Design review of the part built by this model. Coordinates are the model's own, in mm. Face numbers are marked on the shaded views. A direction names the side the tool comes from. Give positions to 0.01 mm unless a question says otherwise; leave off trailing zeros. Order: outer loops, then holes, each group sorted by start corner. A loop starts at its lowest first (then second) coordinate and runs counter-clockwise, first axis right, second up. Notation, with made-up numbers: (11.5, 53.5) - (48.5, 53.5) arc R29 ccw to (48.5, 85.5) - close; hole circle Ø6 at (-1.5, 80). An arc over 180 degrees is marked (long way). Write each question's results on one line, items separated by ' | '. Start each with the question number.
```python
from build123d import *
from build123d import SkipClean  # not in build123d's __all__

# Parameters (mm, degrees)
F0_R     = 50.8
F0_R_2   = 6.35
F0_R_3   = 19.05
F1_DEPTH = 12.7
F2_R     = 25.4
F3_DEPTH = 76.2
F4_R     = 50.8
F4_R_2   = 6.35
F4_R_3   = 19.05
F5_DEPTH = 12.7
F6_R     = 19.05
F7_DEPTH = 76.2


# Not quite as in the source:
# - a feature names something its author has since deleted; it is built from what else it names


with BuildPart() as f1:
    # F0 (on Front) → F1 (new body)
    with BuildSketch(Plane.XZ):
        Circle(F0_R)
        with Locations((-28.575, -28.575)):
            Circle(F0_R_2, mode=Mode.SUBTRACT)
        Circle(F0_R_3, mode=Mode.SUBTRACT)
        with Locations((28.575, -28.575)):
            Circle(F0_R_2, mode=Mode.SUBTRACT)
        with Locations((-28.575, 28.575)):
            Circle(F0_R_2, mode=Mode.SUBTRACT)
        with Locations((28.575, 28.575)):
            Circle(F0_R_2, mode=Mode.SUBTRACT)
    extrude(amount=F1_DEPTH)

    # F2 (on face) → F3 (join)
    with BuildSketch(Plane(origin=(0, 0, 0), x_dir=(-1, 0, 0), z_dir=(0, 1, 0))):
        Circle(F2_R)
    extrude(amount=F3_DEPTH)

    # F4 (on face) → F5 (join)
    with BuildSketch(Plane(origin=(0, 76.2, 0), x_dir=(-1, 0, 0), z_dir=(0, 1, 0))):
        Circle(F4_R)
        with Locations((-28.575, -28.575)):
            Circle(F4_R_2, mode=Mode.SUBTRACT)
        Circle(F4_R_3, mode=Mode.SUBTRACT)
        with Locations((28.575, -28.575)):
            Circle(F4_R_2, mode=Mode.SUBTRACT)
        with Locations((-28.575, 28.575)):
            Circle(F4_R_2, mode=Mode.SUBTRACT)
        with Locations((28.575, 28.575)):
            Circle(F4_R_2, mode=Mode.SUBTRACT)
    extrude(amount=F5_DEPTH)

    # F6 (on face) → F7 (cut)
    with BuildSketch(Plane(origin=(0, 76.2, 0), x_dir=(-1, 0, 0), z_dir=(0, 1, 0))):
        Circle(F6_R)
    with SkipClean():  # cleaning this boolean's faces spoils the solid; the shape is the same uncleaned
        extrude(amount=-F7_DEPTH, mode=Mode.SUBTRACT)


solid = f1.part
```
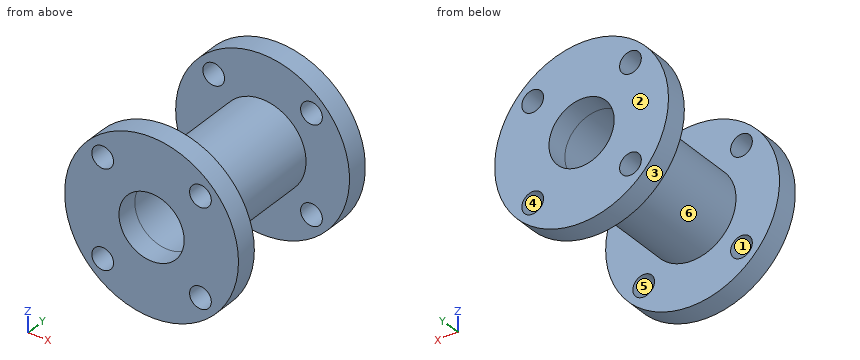
Q1. Machinability: for the marked faces 5 and 6, which of the approach directions +Z, -Z, +X, -X, +Y, -Y give a long, thin tool a straight path to every point of the face, cutting with its end or side? Answer none if there is none.
Q2. Add section A-A (z = 0). Give the boundary of the cut face in (x, y).
Q3. Add section C-C (x = -5). Give the boundary of the cut face in (y, z), plus the area to 3 significant figures.
Q4. Add section B-B (x = 31). Give the boundary of the cut face in (y, z).
Q5. Insertion check: pin 1 Ø20.5 at (x, z) = (28.575, -28.575) entering from +Y; pin 2 Ø10 at (x, z) = (28.575, -28.575) entering from +Y; pin 3 Ø8 at (y, z) = (-1, -23) entering from -X; pin 4 Ø8 at (x, y) = (1.5, 24.5) entering from -Z. Each pin has a flat end and moves straight along its axis. Give the tip position at first contact, or say it passes through.
Q6. For line 1 (Z direction, x = 0, y = 57); line 2 (Z direction, x = -23.5, y = -3); line 3 (Y direction, x = 4.5, z = -45.5), list the stretches that pass through material, from the lowest coordinate up. Write a range as [from, to].
Q7. Add section D-D (y = 2.5). Give the boundary of the cut face in (x, z), plus the area to 3 significant figures.
Q8. Draft analysis for pull direction Z (two halves, no side actions). For the marked faces 1, 2, 3 and 4, state which applies: pulls with the +Z half, pulls with the -Z half, needs draft (parallel to the pull), parting line crosses it, or undercut.
Verdict:
1) face 5: +Y, -Y | face 6: none
2) outline: (-50.8, -12.7) - (-19.05, -12.7) - (-19.05, 88.9) - (-50.8, 88.9) - (-50.8, 76.2) - (-25.4, 76.2) - (-25.4, 0) - (-50.8, 0) - close; (19.05, -12.7) - (50.8, -12.7) - (50.8, 0) - (25.4, 0) - (25.4, 76.2) - (50.8, 76.2) - (50.8, 88.9) - (19.05, 88.9) - close
3) outline: (-12.7, -50.55) - (0, -50.55) - (0, -24.9) - (76.2, -24.9) - (76.2, -50.55) - (88.9, -50.55) - (88.9, -18.38) - (-12.7, -18.38) - close; (-12.7, 18.38) - (88.9, 18.38) - (88.9, 50.55) - (76.2, 50.55) - (76.2, 24.9) - (0, 24.9) - (0, 50.55) - (-12.7, 50.55) - close | area: 2,630 mm2
4) outline: (-12.7, -40.24) - (0, -40.24) - (0, -34.44) - (-12.7, -34.44) - close; (-12.7, -22.71) - (0, -22.71) - (0, 22.71) - (-12.7, 22.71) - close; (-12.7, 34.44) - (0, 34.44) - (0, 40.24) - (-12.7, 40.24) - close; (76.2, -40.24) - (88.9, -40.24) - (88.9, -34.44) - (76.2, -34.44) - close; (76.2, -22.71) - (88.9, -22.71) - (88.9, 22.71) - (76.2, 22.71) - close; (76.2, 34.44) - (88.9, 34.44) - (88.9, 40.24) - (76.2, 40.24) - close
5) pin 1: stops at y = 88.9 | pin 2: passes through | pin 3: stops at x = -47.11 | pin 4: stops at z = -25.4
6) line 1: z = [-25.4, -19.05], [19.05, 25.4] | line 2: z = [-45.04, -32.39], [-24.76, 24.76], [32.39, 45.04] | line 3: y = [-12.7, 0], [76.2, 88.9]
7) outline: circle Ø50.8 at (0, 0); hole circle Ø38.1 at (0, 0) | area: 887 mm2
8) face 1: undercut | face 2: needs draft | face 3: parting line crosses it | face 4: undercut
